from build123d import *

# Parameters (mm, degrees)
SKETCH1_W           = 75
SKETCH1_H           = 40
SKETCH1_R           = 2.5
SKETCH1_R_2         = 1.5
BOSS_EXTRUDE1_DEPTH = 3.175
SKETCH2_R           = 175
CUT_EXTRUDE1_DEPTH  = 3.175
FILLET1_R           = 3
SKETCH3_R           = 5
CUT_EXTRUDE2_DEPTH  = 3.175


with BuildPart() as part:
    # Sketch1 → Boss-Extrude1 (new body)
    with BuildSketch(Plane.XY):
        Rectangle(SKETCH1_W, SKETCH1_H)
        with Locations((-32.5, 15)):
            Circle(SKETCH1_R, mode=Mode.SUBTRACT)
        with Locations((32.5, 15)):
            Circle(SKETCH1_R, mode=Mode.SUBTRACT)
        with Locations((32.5, -15)):
            Circle(SKETCH1_R, mode=Mode.SUBTRACT)
        with Locations((-32.5, -15)):
            Circle(SKETCH1_R, mode=Mode.SUBTRACT)
        with Locations((-8.75, 8.75)):
            Circle(SKETCH1_R_2, mode=Mode.SUBTRACT)
        with Locations((8.75, 8.75)):
            Circle(SKETCH1_R_2, mode=Mode.SUBTRACT)
        with Locations((8.75, -8.75)):
            Circle(SKETCH1_R_2, mode=Mode.SUBTRACT)
        with Locations((-8.75, -8.75)):
            Circle(SKETCH1_R_2, mode=Mode.SUBTRACT)
    extrude(amount=BOSS_EXTRUDE1_DEPTH)

    # Sketch2 → Cut-Extrude1 (cut)
    with BuildSketch(Plane.XY.offset(3.175)):
        with Locations((0, 190.93492914)):
            Circle(SKETCH2_R)
        with Locations((0, -190.93492914)):
            Circle(SKETCH2_R)
    extrude(amount=-CUT_EXTRUDE1_DEPTH, mode=Mode.SUBTRACT)

    # Fillet1
    fillet1_edges = [part.edges().sort_by_distance(p)[0] for p in [
        (-37.5, 20, 1.5875),
        (37.5, 20, 1.5875),
        (37.5, -20, 1.5875),
        (-37.5, -20, 1.5875),
    ]]
    fillet(fillet1_edges, radius=FILLET1_R)

    # Sketch3 → Cut-Extrude2 (cut)
    with BuildSketch(Plane.XY.offset(3.175)):
        Circle(SKETCH3_R)
    extrude(amount=-CUT_EXTRUDE2_DEPTH, mode=Mode.SUBTRACT)


solid = part.part
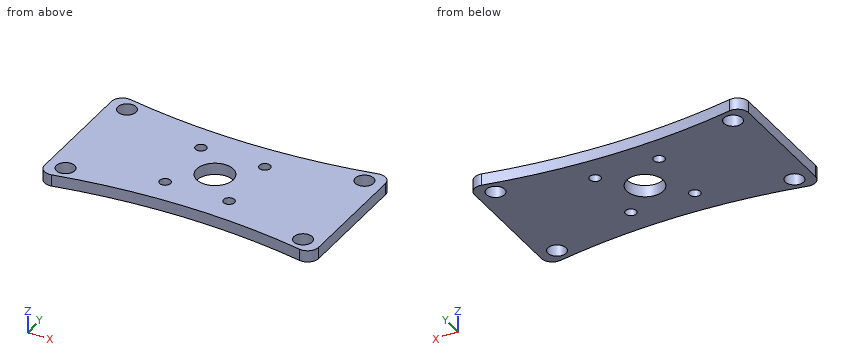
Can you work these out from the model? Positions are in its coordinate system, mm. Round coordinates to 2 decimals unless told otherwise and drop trailing zeros. Write each loop counter-clockwise with the first axis right and the second up, starting at its lowest first coordinate (ties: lowest second). Pieces come first, ordered by that corner, then holes. Notation, with made-up numbers: (-20.5, 66.25) -> (19.5, 66.25) arc R18 cw to (19.5, 91.25) -> close; hole circle Ø5 at (-1, 43). An arc over 180 degrees is marked (long way). Use one line per item in the form item = value. Start each with the question number.
Q1. Imagine slicing it at D-D (x = 0). Please give me the cut outline in (y, z) (3 decimals).
Q2. If I drill on probe 1 along Y at (x, z) = (32.5, 1.95); probe 2 along Y at (x, z) = (-8.75, 1.8); probe 3 along X at (y, z) = (-3, 0.65), over which ranges is the centre line in solid material (lowest first)? Write a range as [from, to].
Q3. Imagine slicing it at B-B (z = 1.1). Count the separate pieces of the cut face and the enclosed holes in it, then the cut area to 3 significant figures.
Q4. I'm going to push flat-ended pins straight in: P1, Ø1, axis at x = 29, z = 1.5, coming from the +Y side; P2, Ø9, axis at x = 0, y = 0, coming from the -Z side. Where does each tip first touch, or does it pass through?
Q5. Imagine slicing it at C-C (x = 9). Please give me the cut outline in (y, z) (3 decimals), then the cut area to 3 significant figures.
Q6. Imagine slicing it at A-A (y = 15). Please give me the cut outline in (x, z) (3 decimals).
Worked out:
q1.outline = (-15.935, 0) -> (-5, 0) -> (-5, 3.175) -> (-15.935, 3.175) -> close; (5, 0) -> (15.935, 0) -> (15.935, 3.175) -> (5, 3.175) -> close
q2.probe_1 = [-18.98, -17.5], [-12.5, 12.5], [17.5, 18.98]
q2.probe_2 = [-16.15, -10.25], [-7.25, 7.25], [10.25, 16.15]
q2.probe_3 = [-37.5, -4], [4, 37.5]
q3.separate_pieces = 1
q3.enclosed_holes = 9
q3.area = 2,390 mm^2
q4.P1 = 18.44
q4.P2 = through
q5.outline = (-16.167, 0) -> (-10.229, 0) -> (-10.229, 3.175) -> (-16.167, 3.175) -> close; (-7.271, 0) -> (7.271, 0) -> (7.271, 3.175) -> (-7.271, 3.175) -> close; (10.229, 0) -> (16.167, 0) -> (16.167, 3.175) -> (10.229, 3.175) -> close
q5.area = 83.9 mm^2
q6.outline = (-37.5, 0) -> (-35, 0) -> (-35, 3.175) -> (-37.5, 3.175) -> close; (-30, 0) -> (30, 0) -> (30, 3.175) -> (-30, 3.175) -> close; (35, 0) -> (37.5, 0) -> (37.5, 3.175) -> (35, 3.175) -> close
